Part print with two shaded views. Sizes in mm from the minimum x, y, z corner. A direction names the side the tool comes from. Coordinates: 2 decimals unless noted, no trailing zeros. Write each loop counter-clockwise with the first axis right and the second up, starting at its lowest first coordinate (ties: lowest second). Pieces come first, ordered by that corner, then holes. Notation, with made-up numbers: (87, 39) - (122, 39) arc R20 ccw to (122, 66) - close; hole circle Ø6 at (41.5, 84). An arc over 180 degrees is marked (long way). One line per question, with ' | ' between items. Start each with the question number.
1. Flat gauge pins, fed straight in: P1, Ø4, axis at x = 30, z = 4, coming from the -Y side; P2, Ø5, axis at x = 1.5, z = 4, coming from the +Y side; P3, Ø2, axis at y = 21.5, z = 9, coming from the -X side. Where does each tip first touch, or does it go through?
2. Which spindle directions (+Z, -Z, +X, -X, +Y, -Y) get a long thin tool onto all of the face, cutting with end or side? Do the marked faces 1, 2, 3 and 4. Say none if no direction does.
3. Band-saw the part on C-C, the plane x = 27. Write the cut outline in (y, z).
4. Probe line 1 (X direction, y = 4.5, z = 9); line 2 (Y direction, x = 27.5, z = 1.25); line 3 (Y direction, x = 31.5, z = 4.5). List the from-to ranges inside material, lowest first.
5. Band-saw the part on B-B, the plane y = 21.25. Write the cut outline in (x, z), then the cut area to 3 significant figures.
6. Band-saw the part on A-A, the plane z = 10.5. Write the cut outline in (x, y).
7. Band-saw the part on D-D, the plane z = 3.5. Write the cut outline in (x, y), then the cut area to 3 significant figures.
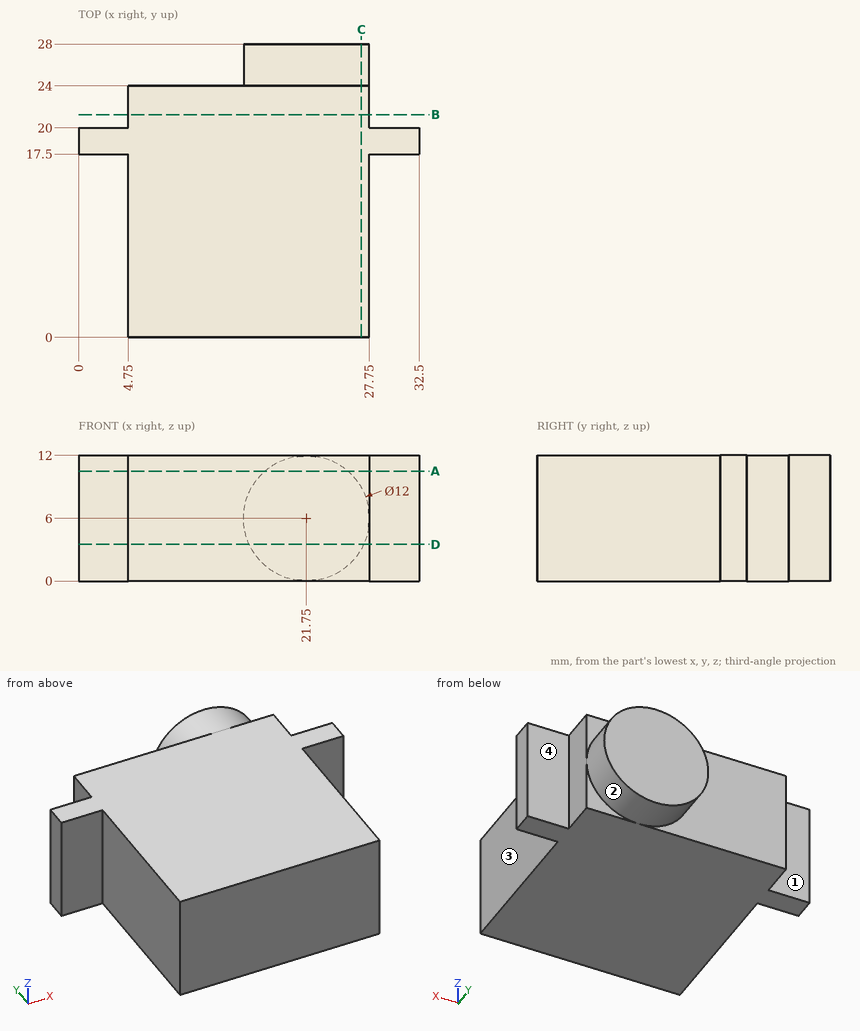
Filled in:
1) P1: stops at y = 17.5 | P2: stops at y = 20 | P3: stops at x = 4.75
2) face 1: +Z, -Z, -X, +Y | face 2: +Y | face 3: +Z, -Z, +X, -Y | face 4: +Z, -Z, +X, +Y
3) outline: (0, 0) - (24, 0) - (24, 3.1) - (28, 3.1) - (28, 8.9) - (24, 8.9) - (24, 12) - (0, 12) - close
4) line 1: x = 4.75 to 27.75 | line 2: y = 0 to 24 | line 3: y = 17.5 to 20
5) outline: (4.75, 0) - (27.75, 0) - (27.75, 12) - (4.75, 12) - close | area: 276 mm²
6) outline: (0, 17.5) - (4.75, 17.5) - (4.75, 0) - (27.75, 0) - (27.75, 17.5) - (32.5, 17.5) - (32.5, 20) - (27.75, 20) - (27.75, 24) - (25.72, 24) - (25.72, 28) - (17.78, 28) - (17.78, 24) - (4.75, 24) - (4.75, 20) - (0, 20) - close
7) outline: (0, 17.5) - (4.75, 17.5) - (4.75, 0) - (27.75, 0) - (27.75, 17.5) - (32.5, 17.5) - (32.5, 20) - (27.75, 20) - (27.75, 24) - (27.2, 24) - (27.2, 28) - (16.3, 28) - (16.3, 24) - (4.75, 24) - (4.75, 20) - (0, 20) - close | area: 619 mm²
